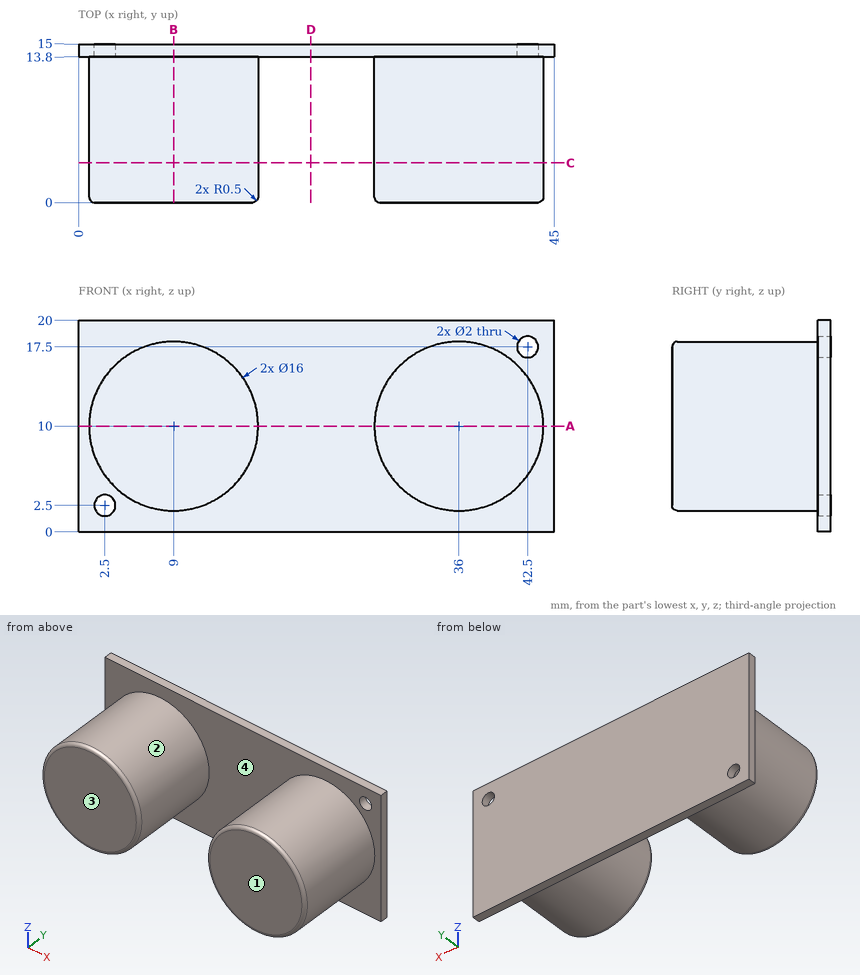
Source: three-view drawing plus pictorial views. Frame: mm from the lowest corner of the part. A direction names the side the tool comes from. Give positions to 0.01 mm unless a question says otherwise; leave off trailing zeros. Write each loop counter-clockwise with the first axis right and the second up, starting at its lowest first coordinate (ties: lowest second). Pieces come first, ordered by that corner, then holes. Notation, with made-up numbers: (28, -28) - (69, -28) arc R23 ccw to (69, 6) - close; hole circle Ø1 at (-28, -5). An arc over 180 degrees is marked (long way). Write item = value, one per line. Start each with the question number.
1. Section query C-C, the plane y = 3.75. Output: boundary loops of the cut face in (x, z), then the cut area to 3 significant figures.
2. Section query A-A, the plane z = 10. Output: boundary loops of the cut face in (x, y), then the cut area to 3 significant figures.
3. Section query D-D, the plane x = 22. Output: boundary loops of the cut face in (y, z).
4. Mould query, pull axis X, two halves, no side actions, for the marked faces 1 and 2. Classes: released by +X, released by -X, zero draft, split by the parting line, or undercut.
5. First-contact query: pin 1 Ø5 at (y, z) = (8, 7.5) entering from +X; pin 2 Ø2.5 at (x, z) = (42.5, 17.5) entering from -Y; pin 3 Ø2 at (y, z) = (6.5, 6.5) entering from +X. Flat tips, straight axial feed; report the tip coordinate or a pass-through.
6. Section query B-B, the plane x = 9. Output: boundary loops of the cut face in (y, z), then the cut area to 3 significant figures.
7. Ray query, L1, parallel to Z at x = 2.5, y = 14.2; L2, parallel to Z at x = 42.5, y = 14.6; L3, parallel to Y at x = 13, z = 19. Return the intervals inside material, ascending.
8. Access query for the marked faces 3 and 4. Directions: +Z, -Z, +X, -X, +Y, -Y. A direction counts if a zero-diameter tool reaches every point of the face in a straight line with its end or side. Return the directions, or none.
Check sheet entries:
q1.outline = circle Ø16 at (9, 10); circle Ø16 at (36, 10)
q1.area = 402 mm2
q2.outline = (0, 13.8) - (1, 13.8) - (1, 0.5) arc R0.5 ccw to (1.5, 0) - (16.5, 0) arc R0.5 ccw to (17, 0.5) - (17, 13.8) - (28, 13.8) - (28, 0.5) arc R0.5 ccw to (28.5, 0) - (43.5, 0) arc R0.5 ccw to (44, 0.5) - (44, 13.8) - (45, 13.8) - (45, 15) - (0, 15) - close
q2.area = 495 mm2
q3.outline = (13.8, 0) - (15, 0) - (15, 20) - (13.8, 20) - close
q4.face_1 = zero draft
q4.face_2 = undercut
q5.pin_1 = 44
q5.pin_2 = 13.8
q5.pin_3 = 43.6
q6.outline = (0, 2.5) arc R0.5 ccw to (0.5, 2) - (13.8, 2) - (13.8, 0) - (15, 0) - (15, 20) - (13.8, 20) - (13.8, 18) - (0.5, 18) arc R0.5 ccw to (0, 17.5) - close
q6.area = 245 mm2
q7.L1 = 0 to 1.5, 3.5 to 20
q7.L2 = 0 to 16.5, 18.5 to 20
q7.L3 = 13.8 to 15
q8.face_3 = +Z, -Z, +X, -X, -Y
q8.face_4 = -Y
